from build123d import *

# Parameters (mm, degrees)
F0_R     = 63.5
F2_DEPTH = 50.8
F1_R     = 12.7
F3_DEPTH = 50.8
F4_R     = 12.7
F5_DEPTH = 79.50153
F6_R     = 5.08
F7_R     = 5.08


with BuildPart() as f2:
    # F0 (on Front) → F2 (new body)
    with BuildSketch(Plane.XZ):
        Circle(F0_R)
    extrude(amount=F2_DEPTH)

    # F1 (on face) → F3 (cut)
    with BuildSketch(Plane.XZ):
        Circle(F1_R)
    extrude(amount=F3_DEPTH, mode=Mode.SUBTRACT)

    # F4 (on Front) → F5 (join, symmetric)
    with BuildSketch(Plane.XZ):
        Circle(F4_R)
    extrude(amount=F5_DEPTH, both=True)

    # F6
    f6_edges = [f2.edges().sort_by_distance(p)[0] for p in [
        (-63.5, -50.8, 0),
    ]]
    fillet(f6_edges, radius=F6_R)

    # F7
    f7_edges = [f2.edges().sort_by_distance(p)[0] for p in [
        (-63.5, 0, 0),
    ]]
    fillet(f7_edges, radius=F7_R)


solid = f2.part
The model under review builds one solid part; all positions refer to its coordinate system, in mm. A direction names the side the tool comes from. Give positions to 0.01 mm unless a question says otherwise; leave off trailing zeros. Loops run counter-clockwise (first coordinate to the right, second up) from the corner with the lowest first, then second, coordinate; pieces in that order, holes last. Notation, with made-up numbers: (82, 68) -> (87, 68) arc R5 cw to (87, 76) -> close; hole circle Ø1 at (24, 10.25). An arc over 180 degrees is marked (long way). Answer as a JSON object with one key per item and string values. Group by question number.
Q1. Take a section at A-A (x = 0). Write out the cut boundary in (y, z).
Q2. Take a section at B-B (z = 0). Write out the cut boundary in (x, y), plus the area to 3 significant figures.
Q3. Tool access review of faces 1 (the cylindrical face through (-2.75, -65.35, -12.4)), 2 (the flat face through (0, -79.502, 0)), 3 (the cylindrical face through (-2.75, 39.19, -12.4)): name each direction out of +Z, -Z, +X, -X, +Y, -Y from which nothing blocks a thin tool from reaching the whole face with its end or side.
Q4. Insertion check: pin 1 (5 mm diameter, centred on x = 26.5, z = 18.5, fed in from -Y); pin 2 (5 mm diameter, centred on y = -52.5, z = -17, fed in from -X); pin 3 (8 mm diameter, centred on y = 52.5, z = -11, fed in from -X). Each pin has a flat end and moves straight along its axis. Give the tip position at first contact, or say it passes through.
Q5. Wall thickness on line 1 along Y through (x, z) = (9.5, 15); line 2 along Z through (x, y) = (0, 2); line 3 along Z through (x, y) = (-4.5, -58): over which ranges is each line inside the solid? List them lowest first.
Answer below:
{
 "1": {"outline": "(-79.5, -12.7) -> (-50.8, -12.7) -> (-50.8, -58.42) arc R5.08 ccw to (-45.72, -63.5) -> (-5.08, -63.5) arc R5.08 ccw to (0, -58.42) -> (0, -12.7) -> (79.5, -12.7) -> (79.5, 12.7) -> (0, 12.7) -> (0, 58.42) arc R5.08 ccw to (-5.08, 63.5) -> (-45.72, 63.5) arc R5.08 ccw to (-50.8, 58.42) -> (-50.8, 12.7) -> (-79.5, 12.7) -> close"},
 "2": {"outline": "(-63.5, -45.72) arc R5.08 ccw to (-58.42, -50.8) -> (-12.7, -50.8) -> (-12.7, -79.5) -> (12.7, -79.5) -> (12.7, -50.8) -> (58.42, -50.8) arc R5.08 ccw to (63.5, -45.72) -> (63.5, -5.08) arc R5.08 ccw to (58.42, 0) -> (12.7, 0) -> (12.7, 79.5) -> (-12.7, 79.5) -> (-12.7, 0) -> (-58.42, 0) arc R5.08 ccw to (-63.5, -5.08) -> close", "area": "9,180 mm2"},
 "3": {"face 1": "-Y", "face 2": "+Z, -Z, +X, -X, -Y", "face 3": "+Y"},
 "4": {"pin 1": "stops at y = -50.8", "pin 2": "stops at x = -58.81", "pin 3": "stops at x = -10.6"},
 "5": {"line 1": "y = -50.8 to 0", "line 2": "z = -12.7 to 12.7", "line 3": "z = -11.88 to 11.88"}
}
